```python
from build123d import *

# Parameters (mm, degrees)
BOSS_EXTRUDE1_DEPTH = 5
SKETCH2_R           = 2
CUT_EXTRUDE1_DEPTH  = 6


with BuildPart() as part:
    # Sketch1 → Boss-Extrude1 (new body)
    with BuildSketch(Plane.XY):
        with BuildLine():
            Line((-19.5, 0), (19.5, 0))
            ThreePointArc((19.5, 0), (20.914213562, 0.585786438), (21.5, 2))
            Line((21.5, 2), (21.5, 10.5))
            ThreePointArc((21.5, 10.5), (21.792893219, 11.207106781), (22.5, 11.5))
            Line((22.5, 11.5), (24.5, 11.5))
            ThreePointArc((24.5, 11.5), (25.207106781, 11.207106781), (25.5, 10.5))
            Line((25.5, 10.5), (25.5, -18.5))
            ThreePointArc((25.5, -18.5), (25.207106781, -19.207106781), (24.5, -19.5))
            Line((24.5, -19.5), (22.5, -19.5))
            ThreePointArc((22.5, -19.5), (21.792893219, -19.207106781), (21.5, -18.5))
            Line((21.5, -18.5), (21.5, -10))
            ThreePointArc((21.5, -10), (20.914213562, -8.585786438), (19.5, -8))
            Line((19.5, -8), (-19.5, -8))
            ThreePointArc((-19.5, -8), (-20.914213562, -7.414213562), (-21.5, -6))
            Line((-21.5, -6), (-21.5, -2))
            ThreePointArc((-21.5, -2), (-20.914213562, -0.585786438), (-19.5, 0))
        make_face()
    extrude(amount=BOSS_EXTRUDE1_DEPTH)

    # Sketch2 → Cut-Extrude1 (cut, through all)
    with BuildSketch(Plane.XY.offset(5)):
        with Locations((-13.5, -4)):
            Circle(SKETCH2_R)
        with Locations((18.5, -4)):
            Circle(SKETCH2_R)
    extrude(amount=-CUT_EXTRUDE1_DEPTH, mode=Mode.SUBTRACT)


solid = part.part
```
Input: part model. Units: mm. Frame: model coordinates. A direction names the side the tool comes from. Give positions to 0.01 mm unless a question says otherwise; leave off trailing zeros. Order: outer loops, then holes, each group sorted by start corner. A loop starts at its lowest first (then second) coordinate and runs counter-clockwise, first axis right, second up. Notation, with made-up numbers: (-39.5, 58.25) - (-2.5, 58.25) arc R21 ccw to (-2.5, 95.25) - close; hole circle Ø8 at (85, -14). An arc over 180 degrees is marked (long way). Use a Markdown table: item, result.
(1) Section query B-B (x = -13.5). Output: boundary loops of the cut face in (y, z).
Computed values:
| item | result |
|---|---|
| outline | (-8, 0) - (-6, 0) - (-6, 5) - (-8, 5) - close; (-2, 0) - (0, 0) - (0, 5) - (-2, 5) - close |
(2) Section query A-A (y = -4). Output: boundary loops of the cut face in (x, z).
Computed values:
| item | result |
|---|---|
| outline | (-21.5, 0) - (-15.5, 0) - (-15.5, 5) - (-21.5, 5) - close; (-11.5, 0) - (16.5, 0) - (16.5, 5) - (-11.5, 5) - close; (20.5, 0) - (25.5, 0) - (25.5, 5) - (20.5, 5) - close |
(3) Line query: line 1 (Y direction, x = -13.5, z = 3.5); line 2 (Y direction, x = 12, z = 2.3); line 3 (X direction, y = -3.5, z = 3.3). Output: solid intervals per line, ascending. Write a range as from..to.
Computed values:
| item | result |
|---|---|
| line 1 | y = -8..-6, -2..0 |
| line 2 | y = -8..0 |
| line 3 | x = -21.5..-15.44, -11.56..16.56, 20.44..25.5 |
(4) Pin query (flat end, axial travel): pin 1 (6.5 mm diameter, centred on x = 18.5, y = -4, fed in from +Z); pin 2 (1.5 mm diameter, centred on x = 5.5, z = 3, fed in from +Y); pin 3 (1 mm diameter, centred on y = -10, z = 1.5, fed in from -X); pin 4 (1.5 mm diameter, centred on x = -7, z = 1.5, fed in from -Y). Return the tip coordinate at first contact, or that it passes through.
Computed values:
| item | result |
|---|---|
| pin 1 | stops at z = 5 |
| pin 2 | stops at y = 0 |
| pin 3 | stops at x = 21.44 |
| pin 4 | stops at y = -8 |
(5) Section query D-D (y = -12). Output: boundary loops of the cut face in (x, z), then the cut area to 3 significant figures.
Computed values:
| item | result |
|---|---|
| outline | (21.5, 0) - (25.5, 0) - (25.5, 5) - (21.5, 5) - close |
| area | 20.0 mm2 |
(6) Access query for faces 1 (the flat face through (21.5, -14, 2)), 2 (the flat face through (8, -4, 5)), 3 (the flat face through (21.5, 6, 2)). Directions: +Z, -Z, +X, -X, +Y, -Y. A direction counts if a zero-diameter tool reaches every point of the face in a straight line with its end or side. Return the directions, or none.
Computed values:
| item | result |
|---|---|
| face 1 | +Z, -Z, -X, -Y |
| face 2 | +Z, +X, -X, +Y, -Y |
| face 3 | +Z, -Z, -X, +Y |
(7) Draft query along X for faces 4 (the cylindrical face through (20.93, -8.6, 2.46)), 5 (the cylindrical face through (-15.1, -5.2, 2.5)), 6 (the flat face through (23, 11.5, 2)). Return one class per face: released by +X, released by -X, zero draft, split by the parting line, or undercut.
Computed values:
| item | result |
|---|---|
| face 4 | released by -X |
| face 5 | undercut |
| face 6 | zero draft |
(8) Section query C-C (z = 1.1). Output: boundary loops of the cut face in (x, y).
Computed values:
| item | result |
|---|---|
| outline | (-21.5, -6) arc R2 ccw to (-19.5, -8) - (19.5, -8) arc R2 cw to (21.5, -10) - (21.5, -18.5) arc R1 ccw to (22.5, -19.5) - (24.5, -19.5) arc R1 ccw to (25.5, -18.5) - (25.5, 10.5) arc R1 ccw to (24.5, 11.5) - (22.5, 11.5) arc R1 ccw to (21.5, 10.5) - (21.5, 2) arc R2 cw to (19.5, 0) - (-19.5, 0) arc R2 ccw to (-21.5, -2) - close; hole circle Ø4 at (-13.5, -4); hole circle Ø4 at (18.5, -4) |
